Autodesk Inventor part; units mm, degrees
ref_plane "YZ Plane" through (0, 0, 0) normal (1, 0, 0) x (0, 1, 0)
ref_plane "XZ Plane" through (0, 0, 0) normal (0, 1, 0) x (-1, 0, 0)
ref_plane "XY Plane" through (0, 0, 0) normal (0, 0, 1) x (1, 0, 0)
sketch "Sketch1" plane through (0, 0, 0) normal (1, 0, 0) x (0, 1, 0)
  circle A0 centre (0.7746, 0) radius 41.021
  point P0 (0, 0)
  dimension "d1" = 82.042
extrude "Extrusion1" add sketch "Sketch1" along normal blind 25.4 draft -22
sketch "Sketch3" plane through (25.4, 0.7746, 0) normal (1, 0, 0) x (0, 0, -1)
  circle A0 centre (0, 0) radius 30.7587
  line L0 (0, 0) -> (-21.4773, 0)
  line L1 (-21.4773, 0) -> (-21.4773, 41.021)
  line L2 (-21.4773, 41.021) -> (0, 41.021)
  line L3 (0, 41.021) -> (0, 0)
  line L4 (30.7587, 0) -> (21.6147, 0)
  line L5 (-21.4773, 41.021) -> (21.6147, 41.021)
  line L6 (21.6147, 41.021) -> (21.6147, -46.8819)
  line L7 (21.6147, -46.8819) -> (-21.4773, -46.8819)
  line L8 (-21.4773, -46.8819) -> (-21.4773, 41.021)
  point P0 (0, -0.7746)
  dimension "d5" = 9.144
extrude "Extrusion2" cut sketch "Sketch3" against normal blind 22.86 contours L6 A0 L8 L0 L3 | A0 L3 L5 L6 | L6 L7 L8 A0 | L3 L0 L1 A0 | A0 L1 L2 L3
sketch "Sketch5" plane through (0, 0.7746, 0) normal (-1, 0, 0) x (0, 0, 1)
  circle A0 centre (0, -0.7746) radius 6.35
  dimension "d13" = 12.7
extrude "Extrusion4" cut sketch "Sketch5" against normal blind 1.27
sketch "Sketch6" plane through (25.4, 0, 0) normal (1, 0, 0) x (0, 0, -1)
  circle A0 centre (-26.5573, 0.7715) radius 1.27
  circle A1 centre (-26.5573, 0.7715) radius 1.27
  point P0 (0, 0)
extrude "Extrusion5" cut sketch "Sketch6" against normal blind 1.27
sketch "Sketch8" plane through (25.4, 0, 0) normal (1, 0, 0) x (0, 0, -1)
  circle A0 centre (26.6947, 0.7715) radius 1.27
  point P0 (0, 0)
extrude "Extrusion7" cut sketch "Sketch8" against normal blind 1.27
properties part number "1st base" material "UHMW, White"
Read the model definition and answer for the solid it produces. Units are mm, in the model's axes. A direction names the side the tool comes from. Give positions to 0.01 mm unless a question says otherwise; leave off trailing zeros. Loops run counter-clockwise (first coordinate to the right, second up) from the corner with the lowest first, then second, coordinate; pieces in that order, holes last. Notation, with made-up numbers: (35.5, 19) -> (80.5, 19) arc R24 ccw to (80.5, 52) -> close; hole circle Ø11 at (35, 33.25). An arc over 180 degrees is marked (long way). Use a Markdown table: item, result.
Q1. Determine the mould class of faces 1 (the face through (1.27, 0, 0)), 2 (the face through (2.54, 1, 0)), 3 (the face through (20.99, -23.21, -21.99)) for opening direction Y: pulls with the +Y half, pulls with the -Y half, needs draft (parallel to the pull), parting line crosses it, or undercut.
Solved:
| item | result |
|---|---|
| face 1 | undercut |
| face 2 | needs draft |
| face 3 | parting line crosses it |
Q2. Section B-B, the plane x = 22.75 is taken. Determine the outline of the cut face in (y, z).
Solved:
| item | result |
|---|---|
| outline | (-22.72, 21.48) -> (24.27, 21.48) arc R31.83 ccw to start; (-22.59, -21.61) arc R31.83 ccw to (24.14, -21.61) -> close |
Q3. Section C-C, the plane x = 15.5 is taken. Determine the outline of the cut face in (y, z).
Solved:
| item | result |
|---|---|
| outline | (-26.55, 21.48) -> (28.1, 21.48) arc R34.76 ccw to start; (-26.45, -21.61) arc R34.76 ccw to (28, -21.61) -> close |
Q4. Each of these flat-tipped pins is pushed along its axis until it touches: pin 1 (12 mm diameter, centred on x = 16, y = -10, fed in from -Z); pin 2 (6 mm diameter, centred on x = 8, z = -20, fed in from +Y); pin 3 (1.5 mm diameter, centred on x = 15.5, y = -29.5, fed in from +Z); pin 4 (11.5 mm diameter, centred on x = 11.5, y = -4.5, fed in from +Z). Where does it stop, or does it pass through?
Solved:
| item | result |
|---|---|
| pin 1 | stops at z = -35.82 |
| pin 2 | stops at y = 33.01 |
| pin 3 | passes through |
| pin 4 | stops at z = 38.43 |
Q5. Find the intervals of material crossed by line 1 along X through (y, z) = (-26.5, 12); line 2 along Z through (x, y) = (20.5, -15.5); line 3 along Z through (x, y) = (5.5, 31.5), in increasing order.
Solved:
| item | result |
|---|---|
| line 1 | x = 0 to 2.54 |
| line 2 | z = -28.41 to -21.61, 21.48 to 28.41 |
| line 3 | z = -23.69 to -21.61, 21.48 to 23.69 |
Q6. Section A-A, the plane z = 0 is taken. Determine the outline of the cut face in (x, y), then the cut area to 3 significant figures.
Solved:
| item | result |
|---|---|
| outline | (0, -40.25) -> (2.54, -39.22) -> (2.54, 40.77) -> (0, 41.8) -> (0, 6.35) -> (1.27, 6.35) -> (1.27, -6.35) -> (0, -6.35) -> close |
| area | 190 mm^2 |
Q7. A tool of negligible diameter and unlimited length cuts with its end or side. For faces 4 (the face through (0, 0, -9)), 5 (the face through (25.4, 0, -25)), 6 (the face through (24.774, 0.827, -25.426)), 7 (the face through (14, 1, -21.615)), 8 (the face through (0.63, -6.2, -1.38)), from which of +Z, -Z, +X, -X, +Y, -Y can it reach the whole face along a straight path? Write none if from no direction.
Solved:
| item | result |
|---|---|
| face 4 | +Z, -Z, -X, +Y, -Y |
| face 5 | +Z, -Z, +X, +Y, -Y |
| face 6 | +X |
| face 7 | +X, +Y, -Y |
| face 8 | -X |
